Geometry: final body of the model. Coordinates: model frame, mm. Face numbers are marked on the shaded views. Give positions to 0.01 mm unless a question says otherwise; leave off trailing zeros. Write each loop counter-clockwise with the first axis right and the second up, starting at its lowest first coordinate (ties: lowest second). Pieces come first, ordered by that corner, then holes. Notation, with made-up numbers: M 33.5,42 L 52.5,42 A22 cw 52.5,71 Z; hole C 71.25,6 d5. An arc over 180 degrees is marked long. One line per question, with ' | ' between items.
from build123d import *


with BuildPart() as f1:
    # F0 (on Front) → F1 (revolve)
    with BuildSketch(Plane.XZ):
        with BuildLine():
            Line((7.62, 7.62), (5.08, 7.62))
            Line((5.08, 7.62), (5.08, 6.985))
            Line((5.08, 6.985), (7.62, 6.985))
            ThreePointArc((7.62, 6.985), (8.813216, 6.669333), (9.694241, 5.804921))
            Line((9.694241, 5.804921), (12.074054, 1.801173))
            ThreePointArc((12.074054, 1.801173), (13.418775, 0.481808), (15.24, 0))
            Line((15.24, 0), (19.05, 0))
            Line((19.05, 0), (19.05, 0.635))
            Line((19.05, 0.635), (15.24, 0.635))
            ThreePointArc((15.24, 0.635), (13.732779, 1.033738), (12.619906, 2.125626))
            Line((12.619906, 2.125626), (10.240094, 6.129374))
            ThreePointArc((10.240094, 6.129374), (9.127221, 7.221262), (7.62, 7.62))
        make_face()
    revolve(axis=Axis((0, 0, 3.02236), (0, 0, 1)))


solid = f1.part
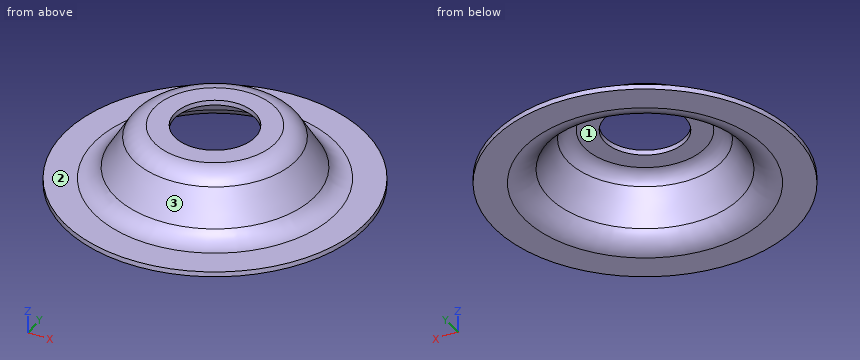
(1) Cut plane B-B, the plane z = 5. Return loops of the section in (x, y).
Working result:
outline: C 0,0 d21.82; hole C 0,0 d20.35
(2) First-contact query: P1, Ø2, axis at x = -6.5, z = 2, coming from the -Y side; P2, Ø2, axis at x = -0.5, z = 2, coming from the +Y side; P3, Ø1, axis at y = 12, z = 4.5, coming from the -X side; P4, Ø2, axis at x = 8.5, z = 4, coming from the +Y side. Flat tips, straight axial feed; report the tip coordinate or a pass-through.
Working result:
P1: stops at y = -12.23 | P2: stops at y = 13.78 | P3: passes through | P4: stops at y = 9.03
(3) Material intervals for L1, parallel to Z at x = -16, y = 0.5 (3 decimals); L2, parallel to Z at x = 6, y = 2.5 (3 decimals); L3, parallel to X at y = -2, z = 4, sorted ascending. Write a range as [from, to].
Working result:
L1: z = [0, 0.635] | L2: z = [6.985, 7.62] | L3: x = [-11.33, -10.58], [10.58, 11.33]
(4) Draft query along Y for the marked faces 1, 2 and 3. Return one class per face: released by +Y, released by -Y, zero draft, split by the parting line, or undercut.
Working result:
face 1: undercut | face 2: zero draft | face 3: split by the parting line
(5) Cut plane A-A, the plane y = 0. Return loops of the section in (x, z) (3 decimals).
Working result:
outline: M -19.05,0 L -15.24,0 A3.683 ccw -12.074,1.801 L -9.694,5.805 A2.413 cw -7.62,6.985 L -5.08,6.985 L -5.08,7.62 L -7.62,7.62 A3.048 ccw -10.24,6.129 L -12.62,2.126 A3.048 cw -15.24,0.635 L -19.05,0.635 Z; M 5.08,6.985 L 7.62,6.985 A2.413 cw 9.694,5.805 L 12.074,1.801 A3.683 ccw 15.24,0 L 19.05,0 L 19.05,0.635 L 15.24,0.635 A3.048 cw 12.62,2.126 L 10.24,6.129 A3.048 ccw 7.62,7.62 L 5.08,7.62 Z
